Here's how the part is built. I have some questions about the finished solid (model axes, mm). A direction names the side the tool comes from. Coordinates: 2 decimals unless noted, no trailing zeros. Write each loop counter-clockwise with the first axis right and the second up, starting at its lowest first coordinate (ties: lowest second). Pieces come first, ordered by that corner, then holes.
Item 1: If I drill on line 1 (Y direction, x = 0, z = 4.75); line 2 (Y direction, x = 0, z = 6.75); line 3 (X direction, y = 0.5, z = 6), over which ranges is the centre line in solid material (lowest first)?
Item 2: If we section it at C-C (x = -26): Please give me the cut outline in (y, z).
Item 3: If we section it at A-A (y = 47.25): Please give me the cut outline in (x, z), then the cut area to 3 significant figures.
Item 4: If we section it at D-D (x = 21): Please give me the cut outline in (y, z).
Item 5: If we section it at B-B (z = 2): Please give me the cut outline in (x, y).
Item 6: We'd pull the mould along Y, two halves only. Please class faces 3 (the face through (-0.54, -2.44, 4.93)), 4 (the face through (-0.84, 137.99, 4.93)), 5 (the face through (9, 51, 0)), 6 (the face through (0.84, -37.99, 4.93)): +Y half, -Y half, draft (parallel to the pull), parting line (faces both ways), or undercut.
Item 7: For faces 1 (the face through (-1.73, 92.19, 2.71)), 2 (the face through (1.846, 96.451, 7.719)), which set-ups out of +Z, -Z, +X, -X, +Y, -Y let a thin tool reach every point of the face, with its end or its side?
Item 8: I'm going to push flat-ended pins straight in: pin 1 Ø1 at (x, z) = (-4, 3) entering from -Y; pin 2 Ø13 at (x, y) = (0, 100) entering from +Z; pin 3 Ø4 at (y, z) = (112.5, 4) entering from -X; pin 4 Ø3 at (x, z) = (5.5, 3.5) entering from +Y. Where does each tip first touch, or does it pass through?
from build123d import *

# Parameters (mm, degrees)
CROQUIS1_R              = 2.5
CROQUIS1_R_2            = 8
CROQUIS1_R_3            = 4
SALIENTE_EXTRUIR1_DEPTH = 10
SALIENTE_EXTRUIR2_START = -4.5
CROQUIS2_R              = 8
CROQUIS2_R_2            = 4
SALIENTE_EXTRUIR2_DEPTH = 4.5


with BuildPart() as part:
    # Croquis1 → Saliente-Extruir1 (new body)
    with BuildSketch(Plane.XY):
        with BuildLine():
            Line((-38, 0), (-38, 100))
            ThreePointArc((-38, 100), (0, 138), (38, 100))
            Line((38, 100), (38, 0))
            ThreePointArc((38, 0), (0, -38), (-38, 0))
        make_face()
        Circle(CROQUIS1_R, mode=Mode.SUBTRACT)
        with Locations((0, 100)):
            Circle(CROQUIS1_R_2, mode=Mode.SUBTRACT)
        with Locations((0, 47.25)):
            Circle(CROQUIS1_R_3, mode=Mode.SUBTRACT)
    extrude(amount=SALIENTE_EXTRUIR1_DEPTH)

    # Croquis2 → Saliente-Extruir2 (add)
    with BuildSketch(Plane.XY.offset(10).offset(SALIENTE_EXTRUIR2_START)):
        with Locations((0, 100)):
            Circle(CROQUIS2_R)
        with Locations((0, 100)):
            Circle(CROQUIS2_R_2, mode=Mode.SUBTRACT)
    extrude(amount=SALIENTE_EXTRUIR2_DEPTH)


solid = part.part
Answer list:
1. line 1: y = -38 to -2.5, 2.5 to 43.25, 51.25 to 92, 108 to 138
1. line 2: y = -38 to -2.5, 2.5 to 43.25, 51.25 to 96, 104 to 138
1. line 3: x = -38 to -2.45, 2.45 to 38
2. outline: (-27.71, 0) - (127.71, 0) - (127.71, 10) - (-27.71, 10) - close
3. outline: (-38, 0) - (-4, 0) - (-4, 10) - (-38, 10) - close; (4, 0) - (38, 0) - (38, 10) - (4, 10) - close
3. area: 680 mm2
4. outline: (-31.67, 0) - (131.67, 0) - (131.67, 10) - (-31.67, 10) - close
5. outline: (-38, 0) arc R38 ccw to (38, 0) - (38, 100) arc R38 ccw to (-38, 100) - close; hole circle Ø16 at (0, 100); hole circle Ø8 at (0, 47.25); hole circle Ø5 at (0, 0)
6. face 3: undercut
6. face 4: +Y half
6. face 5: draft
6. face 6: -Y half
7. face 1: -Z
7. face 2: +Z, -Z
8. pin 1: stops at y = -37.84
8. pin 2: stops at z = 10
8. pin 3: stops at x = -36.52
8. pin 4: stops at y = 137.79
